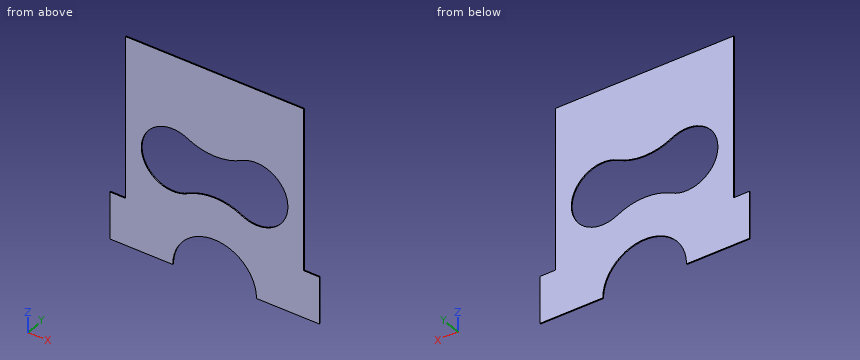
from build123d import *

# Parameters (mm, degrees)
EXTRUSION1_DEPTH = 10


with BuildPart() as part:
    # Esquisse1 → Extrusion1 (new body)
    with BuildSketch(Plane(origin=(0, 0, 0), x_dir=(1, 0, 0), z_dir=(0, 1, 0))):
        with BuildLine():
            Line((2350, 0), (650, 0))
            Line((650, 0), (650, 1550))
            Line((650, 1550), (500, 1550))
            Line((500, 1550), (500, 2000))
            Line((500, 2000), (1100, 2000))
            ThreePointArc((1100, 2000), (1500, 1600), (1900, 2000))
            Line((1900, 2000), (2500, 2000))
            Line((2500, 2000), (2500, 1550))
            Line((2500, 1550), (2350, 1550))
            Line((2350, 1550), (2350, 0))
        make_face()
        with BuildLine():
            ThreePointArc((1241.176470588, 1264.705882353), (800, 1000), (1241.176470588, 735.294117647))
            ThreePointArc((1241.176470588, 735.294117647), (1500, 800), (1758.823529412, 735.294117647))
            ThreePointArc((1758.823529412, 735.294117647), (2200, 1000), (1758.823529412, 1264.705882353))
            ThreePointArc((1758.823529412, 1264.705882353), (1500, 1200), (1241.176470588, 1264.705882353))
        make_face(mode=Mode.SUBTRACT)
    extrude(amount=EXTRUSION1_DEPTH)


solid = part.part
Design review of the part built by this model. Coordinates are the model's own, in mm. Give positions to 0.01 mm unless a question says otherwise; leave off trailing zeros. Loops run counter-clockwise (first coordinate to the right, second up) from the corner with the lowest first, then second, coordinate; pieces in that order, holes last. Notation, with made-up numbers: (-39, 3) - (14, 3) arc R20 cw to (14, 21) - close; hole circle Ø1 at (17.25, 79.5). An arc over 180 degrees is marked (long way). Use CSV: the item, a comma, the result in double quotes. Start each with the question number.
1. Insertion check: P1, Ø1, axis at y = 7.5, z = -1434, coming from the +X side; P2, Ø2, axis at x = 1254.5, y = 8, coming from the -Z side; P3, Ø5, axis at x = 2411, y = 3, coming from the +Z side. Each pin has a flat end and moves straight along its axis. Give the tip position at first contact, or say it passes through.
2. Wall thickness on L1, parallel to Z at x = 1900.5, y = 9.75; L2, parallel to X at y = 5, z = -1172.5; L3, parallel to X at y = 8.5, z = -98.5: over which ranges is each line inside the solid? List them lowest first.
3. Add section A-A (x = 1500). State the section outline as (y, z) points.
4. Add section D-D (z = -416). State the section outline as (x, y) points.
5. Add section B-B (z = -1000). State the section outline as (x, y) points.
6. Add section C-C (y = 6.5). State the section outline as (x, z) points.
Results found:
1,P1,"stops at x = 2350"
1,P2,"stops at z = -1684.98"
1,P3,"stops at z = -1550"
2,L1,"z = -2000 to -1300, -700 to 0"
2,L2,"x = 650 to 854.55, 2145.45 to 2350"
2,L3,"x = 650 to 2350"
3,outline,"(0, -1600) - (10, -1600) - (10, -1200) - (0, -1200) - close; (0, -800) - (10, -800) - (10, 0) - (0, 0) - close"
4,outline,"(650, 0) - (2350, 0) - (2350, 10) - (650, 10) - close"
5,outline,"(650, 0) - (800, 0) - (800, 10) - (650, 10) - close; (2200, 0) - (2350, 0) - (2350, 10) - (2200, 10) - close"
6,outline,"(500, -2000) - (1100, -2000) arc R400 cw to (1900, -2000) - (2500, -2000) - (2500, -1550) - (2350, -1550) - (2350, 0) - (650, 0) - (650, -1550) - (500, -1550) - close; hole (1241.18, -1264.71) arc R550 cw to (1758.82, -1264.71) arc R300 ccw (long way) to (1758.82, -735.29) arc R550 cw to (1241.18, -735.29) arc R300 ccw (long way) to start"
